Drawing for the job (mm, zero at the part's lowest x, y, z). A direction names the side the tool comes from. Coordinates: 2 decimals unless noted, no trailing zeros. Order: outer loops, then holes, each group sorted by start corner. A loop starts at its lowest first (then second) coordinate and runs counter-clockwise, first axis right, second up. Notation, with made-up numbers: (11.25, 28.25) - (38.25, 28.25) arc R26 cw to (38.25, 62.25) - close; hole circle Ø4 at (28, 29.5). An arc over 180 degrees is marked (long way). Put each result on its own line as item: value. Start each with the question number.
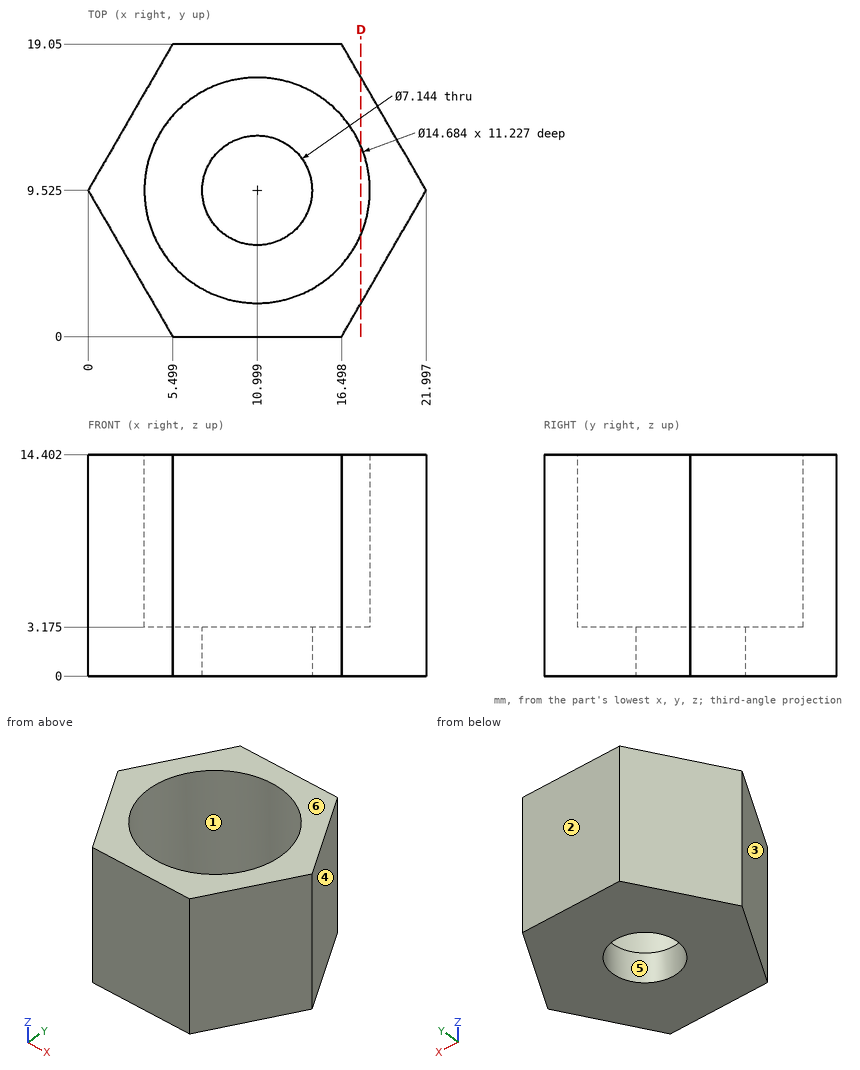
Item 1: 3-axis set-ups, long thin cutter, end or side, ignore diameter. For the marked faces 1 and 2: which of +Z, -Z, +X, -X, +Y, -Y reach the whole face in a straight line?
Item 2: Pull direction Y, two halves, no side cores. Call the marked faces 3, 4, 5 and 6: pulls with the +Y half, pulls with the -Y half, needs draft (parallel to the pull), parting line crosses it, or undercut.
Item 3: Slice it at D-D, the plane x = 17.75. Give the cut face in (y, z) (1 decimal).
Item 4: Wall check: line 1 along Z through (x, y) = (11.5, 4) (1 decimal); line 2 along Y through (x, z) = (5, 10.5) (1 decimal); line 3 along X through (y, z) = (9, 11.75) (1 decimal). Give the ranges that are in metal, low to high.
Item 5: Flat gauge pins, fed straight in: pin 1 Ø2 at (y, z) = (14, 11.5) entering from +X; pin 2 Ø1.5 at (y, z) = (12, 2) entering from -X (1 decimal); pin 3 Ø1.5 at (x, z) = (6.5, 11.5) entering from -Y; pin 4 Ø2 at (y, z) = (2, 6) entering from +X. Where does each tip first touch, or does it go through?
Here are the results:
1. face 1: +Z
1. face 2: +Z, -Z, +X, -X, +Y
2. face 3: pulls with the -Y half
2. face 4: pulls with the +Y half
2. face 5: undercut
2. face 6: needs draft
3. outline: (2.2, 0) - (16.9, 0) - (16.9, 14.4) - (12.4, 14.4) - (12.4, 3.2) - (6.6, 3.2) - (6.6, 14.4) - (2.2, 14.4) - close
4. line 1: z = 0 to 3.2
4. line 2: y = 0.9 to 5.3, 13.8 to 18.2
4. line 3: x = 0.3 to 3.7, 18.3 to 21.7
5. pin 1: stops at x = 19.99
5. pin 2: stops at x = 1
5. pin 3: stops at y = 0
5. pin 4: stops at x = 18.23
